Here's how the part is built. I have some questions about the finished solid (model axes, mm). A direction names the side the tool comes from. Give positions to 0.01 mm unless a question says otherwise; leave off trailing zeros. Write each loop counter-clockwise with the first axis right and the second up, starting at its lowest first coordinate (ties: lowest second). Pieces come first, ordered by that corner, then holes. Notation, with made-up numbers: M 54,78 L 97,78 A12 cw 97,101 Z; hole C 46,-4 d10. An arc over 180 degrees is marked long. Answer as CSV lines item,"result". Start each with the question number.
Q1. For pin 1 (5 mm diameter, centred on x = -12.5, y = 9, fed in from +Z); pin 2 (1.5 mm diameter, centred on x = -3.5, z = -23, fed in from -Y); pin 3 (6 mm diameter, centred on y = -10.5, z = 15.5, fed in from -X), each with a flat end and sliding along its axis, tell me the tip position at first contact or that it passes through.
Q2. Suppose I cut it at A-A (x = 0). Write out the boundary of the cut face in (y, z), then the cut area to 3 significant figures.
Q3. If I drill on line 1 along Z through (x, y) = (13, 8); line 2 along X through (y, z) = (-1, 39); line 3 along X through (y, z) = (8, -6), over which ranges is the centre line in solid material (lowest first)?
Q4. Suppose I cut it at D-D (z = 30). Write out the boundary of the cut face in (x, y).
Q5. Suppose I cut it at C-C (z = 14). Write out the boundary of the cut face in (x, y).
Q6. On a 3-axis mill with a long thin cutter (end or side, diameter ignored), from which of +Z, -Z, +X, -X, +Y, -Y can I reach the whole of each face in a straight line? I mean faces 1 (the flat face through (0, 0, -43.5)), 2 (the cylindrical face through (-1.5, 0.07, 32.99)), 3 (the cylindrical face through (-1.5, 0.07, -35.24)). Say none if no direction works.
```python
from build123d import *

# Parameters (mm, degrees)
SKETCH1_R           = 1.5
BOSS_EXTRUDE1_DEPTH = 43.5
SKETCH4_R           = 16.5
SKETCH4_R_2         = 1.5
BOSS_EXTRUDE2_DEPTH = 50
CHAMFER1_SIZE       = 0.3


with BuildPart() as part:
    # Sketch1 → Boss-Extrude1 (new, symmetric)
    with BuildSketch(Plane.XY):
        Circle(SKETCH1_R)
    extrude(amount=BOSS_EXTRUDE1_DEPTH, both=True)

    # Sketch4 → Boss-Extrude2 (add)
    with BuildSketch(Plane.XY.offset(22.5)):
        Circle(SKETCH4_R)
        Circle(SKETCH4_R_2, mode=Mode.SUBTRACT)
    extrude(amount=-BOSS_EXTRUDE2_DEPTH)

    # Chamfer1
    chamfer1_edges = [part.edges().sort_by_distance(p)[0] for p in [
        (-1.5, 0, -43.5),
        (-1.5, 0, 43.5),
    ]]
    chamfer(chamfer1_edges, length=CHAMFER1_SIZE)


solid = part.part
```
Resolved:
1,pin 1,"z = 22.5"
1,pin 2,"y = -16.27"
1,pin 3,"x = -14.7"
2,outline,"M -16.5,-27.5 L -1.5,-27.5 L -1.5,-43.2 L -1.2,-43.5 L 1.2,-43.5 L 1.5,-43.2 L 1.5,-27.5 L 16.5,-27.5 L 16.5,22.5 L 1.5,22.5 L 1.5,43.2 L 1.2,43.5 L -1.2,43.5 L -1.5,43.2 L -1.5,22.5 L -16.5,22.5 Z"
2,area,"1,760 mm^2"
3,line 1,"-27.5 to 22.5"
3,line 2,"-1.12 to 1.12"
3,line 3,"-14.43 to 14.43"
4,outline,"C 0,0 d3"
5,outline,"C 0,0 d33"
6,face 1,"-Z, +X, -X, +Y, -Y"
6,face 2,"+Z"
6,face 3,"-Z"
